```python
from build123d import *

# Parameters (mm, degrees)
BOSS_EXTRUDE1_DEPTH = 12.7
SKETCH2_R           = 2.5
CUT_EXTRUDE1_DEPTH  = 16.24
SKETCH3_W           = 7.62
SKETCH3_H           = 3.81
CUT_EXTRUDE2_DEPTH  = 81.8409129


with BuildPart() as part:
    # Sketch1 → Boss-Extrude1 (new body)
    with BuildSketch(Plane.XY):
        with BuildLine():
            Line((-40.4204564, 0), (40.4204564, 0))
            Line((40.4204564, 0), (40.4204564, -15.24))
            ThreePointArc((40.4204564, -15.24), (0, -11.830472076), (-40.4204564, -15.24))
            Line((-40.4204564, -15.24), (-40.4204564, 0))
        make_face()
    extrude(amount=BOSS_EXTRUDE1_DEPTH)

    # Sketch2 → Cut-Extrude1 (cut, through all)
    with BuildSketch(Plane(origin=(0, 0, 0), x_dir=(1, 0, 0), z_dir=(0, 1, 0))):
        with Locations((-33.4204564, -6.35)):
            Circle(SKETCH2_R)
        with Locations((33.4204564, -6.35)):
            Circle(SKETCH2_R)
    extrude(amount=-CUT_EXTRUDE1_DEPTH, mode=Mode.SUBTRACT)

    # Sketch3 → Cut-Extrude2 (cut, through all)
    with BuildSketch(Plane(origin=(40.4204564, 0, 0), x_dir=(0, 0, -1), z_dir=(1, 0, 0))):
        with Locations((-6.35, -13.335)):
            Rectangle(SKETCH3_W, SKETCH3_H)
    extrude(amount=-CUT_EXTRUDE2_DEPTH, mode=Mode.SUBTRACT)


solid = part.part
```
Geometry check sheet. Reference: the model listing, model coordinates, mm. A direction names the side the tool comes from. Give positions to 0.01 mm unless a question says otherwise; leave off trailing zeros. Order: outer loops, then holes, each group sorted by start corner. A loop starts at its lowest first (then second) coordinate and runs counter-clockwise, first axis right, second up.
1. Release check for a two-part mould opening along X. For faces 3 (the face through (-1, 0, 6)), 4 (the face through (-40.42, -8, 6)), 5 (the face through (0.57, -11.83, 11.41)) record: pulls with the +X half, pulls with the -X half, needs draft (parallel to the pull), parting line crosses it, or undercut.
2. Access from +Z, -Z, +X, -X, +Y, -Y to the whole of each face (thin tool, end or side, straight path). Record for faces 1 (the face through (0.57, -11.83, 1.25)), 2 (the face through (0.57, -11.67, 2.54)).
3. Section check A-A, the plane y = -5.25. Enter the section's corners in (x, z), and give its area (3 significant figures).
4. Thickness scan on L1, parallel to X at y = -3, z = 6.35; L2, parallel to X at y = -9.75, z = 7.25; L3, parallel to Y at x = -0.5, z = 9.5. Record the ranges inside material, lowest first.
5. Section check B-B, the plane z = 6.35. Enter the section's corners in (x, y), and give its area (3 significant figures).
6. Gauge pin test, flat end, axial feed: pin 1 Ø1.5 at (x, z) = (32, 5) entering from -Y. Record the tip position at first contact, or that the pin passes through.
7. Section check D-D, the plane x = -5. Enter the section's corners in (y, z), and give its area (3 significant figures).
8. Section check C-C, the plane x = 32.5. Enter the section's corners in (y, z), and give its area (3 significant figures).
Values follow:
1. face 3: needs draft
1. face 4: pulls with the -X half
1. face 5: undercut
2. face 1: +Z, -Z, -Y
2. face 2: +X, -X, -Y
3. outline: (-40.42, 0) - (40.42, 0) - (40.42, 12.7) - (-40.42, 12.7) - close; hole circle Ø5 at (-33.42, 6.35); hole circle Ø5 at (33.42, 6.35)
3. area: 987 mm2
4. L1: x = -40.42 to -35.92, -30.92 to 30.92, 35.92 to 40.42
4. L2: x = -40.42 to -35.75, -31.09 to 31.09, 35.75 to 40.42
4. L3: y = -11.43 to 0
5. outline: (-40.42, -11.43) - (-35.92, -11.43) - (-35.92, 0) - (-40.42, 0) - close; (-30.92, -11.43) - (30.92, -11.43) - (30.92, 0) - (-30.92, 0) - close; (35.92, -11.43) - (40.42, -11.43) - (40.42, 0) - (35.92, 0) - close
5. area: 810 mm2
6. pin 1: stops at y = -11.43
7. outline: (-11.88, 0) - (0, 0) - (0, 12.7) - (-11.88, 12.7) - (-11.88, 10.16) - (-11.43, 10.16) - (-11.43, 2.54) - (-11.88, 2.54) - close
7. area: 147 mm2
8. outline: (-14.03, 0) - (0, 0) - (0, 4.03) - (-11.43, 4.03) - (-11.43, 2.54) - (-14.03, 2.54) - close; (-14.03, 10.16) - (-11.43, 10.16) - (-11.43, 8.67) - (0, 8.67) - (0, 12.7) - (-14.03, 12.7) - close
8. area: 105 mm2
